```python
from build123d import *

# Parameters (mm, degrees)
BOSS_EXTRUDE2_DEPTH   = 21.844
BOSS_EXTRUDE2_2_DEPTH = 21.844
SKETCH3_W             = 4.1275
SKETCH3_H             = 39.7002
BOSS_EXTRUDE3_DEPTH   = 1.6002
SKETCH4_W             = 1.6002
SKETCH4_H             = 39.7002
BOSS_EXTRUDE4_DEPTH   = 6.5532
SKETCH5_W             = 23.4442
SKETCH5_H             = 39.7002
BOSS_EXTRUDE5_DEPTH   = 1.6002
BOSS_EXTRUDE6_DEPTH   = 4.7752
SKETCH7_W             = 21.844
SKETCH7_H             = 27.9146
CUT_EXTRUDE1_DEPTH    = 6.35


with BuildPart() as part:
    # Sketch2 → Boss-Extrude2 (new body)
    with BuildSketch(Plane(origin=(0, 0, 0), x_dir=(0, 0, -1), z_dir=(1, 0, 0))):
        Polygon((-8.001, 19.8501), (-8.001, 16.4973), (-6.4135, 16.4973), (-6.4135, 13.9573), (-10.541, 13.9573), (-10.541, 19.8501), align=None)
    extrude(amount=BOSS_EXTRUDE2_DEPTH)



with BuildPart() as body_2:
    # Sketch2 → Boss-Extrude2 2 (new body)
    with BuildSketch(Plane(origin=(0, 0, 0), x_dir=(0, 0, -1), z_dir=(1, 0, 0))):
        Polygon((-6.4135, -16.4973), (-6.4135, -13.9573), (-10.541, -13.9573), (-10.541, -19.8501), (-8.001, -19.8501), (-8.001, -16.4973), align=None)
    extrude(amount=BOSS_EXTRUDE2_2_DEPTH)


with BuildPart() as part_1:
    add(part.part)

    add(body_2.part)  # Boss-Extrude3 merges body 2
    # Sketch3 → Boss-Extrude3 (add)
    with BuildSketch(Plane.ZY):
        with Locations((8.47725, 0)):
            Rectangle(SKETCH3_W, SKETCH3_H)
    extrude(amount=BOSS_EXTRUDE3_DEPTH)

    # Sketch4 → Boss-Extrude4 (add)
    with BuildSketch(Plane(origin=(0, 0, 6.4135), x_dir=(-1, 0, 0), z_dir=(0, 0, -1))):
        with Locations((0.8001, 0)):
            Rectangle(SKETCH4_W, SKETCH4_H)
    extrude(amount=BOSS_EXTRUDE4_DEPTH)

    # Sketch5 → Boss-Extrude5 (add)
    with BuildSketch(Plane(origin=(0, 0, -0.1397), x_dir=(-1, 0, 0), z_dir=(0, 0, -1))):
        with Locations((-10.1219, 0)):
            Rectangle(SKETCH5_W, SKETCH5_H)
    extrude(amount=BOSS_EXTRUDE5_DEPTH)

    # Sketch6 → Boss-Extrude6 (add)
    with BuildSketch(Plane(origin=(0, 19.8501, 0), x_dir=(1, 0, 0), z_dir=(0, 1, 0))):
        Polygon((21.844, -8.001), (0, -8.001), (0, 0.1397), (21.844, 0.1397), (21.844, 1.7399), (-1.6002, 1.7399), (-1.6002, -10.541), (21.844, -10.541), align=None)
    boss_extrude6 = extrude(amount=BOSS_EXTRUDE6_DEPTH)

    # Mirror1: Boss-Extrude6 across plane
    add(boss_extrude6.mirror(Plane.ZX))

    # Sketch7 → Cut-Extrude1 (cut)
    with BuildSketch(Plane.XY.offset(-0.1397)):
        with Locations((10.922, 0)):
            Rectangle(SKETCH7_W, SKETCH7_H)
    extrude(amount=-CUT_EXTRUDE1_DEPTH, mode=Mode.SUBTRACT)


solid = part_1.part
```
Part model, mm, in its own coordinate system. A direction names the side the tool comes from. Coordinates: 2 decimals unless noted, no trailing zeros. Order: outer loops, then holes, each group sorted by start corner. A loop starts at its lowest first (then second) coordinate and runs counter-clockwise, first axis right, second up. Notation, with made-up numbers: (-17, 52) - (-2, 52) arc R24 cw to (-2, 90) - close; hole circle Ø3 at (30.5, 2). An arc over 180 degrees is marked (long way). Return JSON: item names as keys, results as strings. Group by question number.
Item 1: Pull direction Z, two halves, no side cores. Call faces 6 (the face through (-0.5, 0.3, 10.541)), 7 (the face through (11, 15, 6.413)), 8 (the face through (11, 13.957, 8)): pulls with the +Z half, pulls with the -Z half, needs draft (parallel to the pull), parting line crosses it, or undercut.
Item 2: Cut at B-B (y = -15.5). List the corners of the cut face in (x, z).
Item 3: Which spindle directions (+Z, -Z, +X, -X, +Y, -Y) get a long thin tool onto all of the face, cutting with end or side? Do faces 1 (the face through (11, 16.497, 7)), 2 (the face through (11, -19, -0.14)), 3 (the face through (11, -16.497, 7)), 4 (the face through (11, 13.957, -1)), 5 (the face through (21.844, -19, 9)). Say none if no direction does.
Item 4: Cut at D-D (y = -9.5). List the corners of the cut face in (x, z).
Item 5: Cut at C-C (z = -0.75). List the corners of the cut face in (x, y), plus the area to 3 significant figures.
Item 6: Pin check, flat tips, straight feed: pin 1 (3 mm diameter, centred on x = 5.5, z = 5.5, fed in from -Y); pin 2 (12 mm diameter, centred on x = 12.5, y = -5.5, fed in from +Z); pin 3 (0.8 mm diameter, centred on x = 16, z = 7, fed in from +Y). Stop position of each tip, or through.
Item 7: Drill centre lines: probe 1 along Y at (x, z) = (15.5, 7); probe 2 along Z at (x, y) = (4, -14); probe 3 along Z at (x, y) = (17.5, 21). Where is each one in solid material? Low to high. Write a range as from..to.
Item 8: Cut at A-A (x = 3.25). List the corners of the cut face in (y, z).
Check values:
{
 "1": {"face 6": "pulls with the +Z half", "face 7": "undercut", "face 8": "needs draft"},
 "2": {"outline": "(-1.6, -1.74) - (21.84, -1.74) - (21.84, -0.14) - (0, -0.14) - (0, 6.41) - (21.84, 6.41) - (21.84, 10.54) - (-1.6, 10.54) - close"},
 "3": {"face 1": "+X, +Y", "face 2": "+X, +Y, -Y", "face 3": "+X, -Y", "face 4": "+Z, -Z, +X", "face 5": "+Z, -Z, +X, +Y, -Y"},
 "4": {"outline": "(-1.6, -1.74) - (0, -1.74) - (0, 10.54) - (-1.6, 10.54) - close"},
 "5": {"outline": "(-1.6, -24.63) - (21.84, -24.63) - (21.84, -13.96) - (0, -13.96) - (0, 13.96) - (21.84, 13.96) - (21.84, 24.63) - (-1.6, 24.63) - close", "area": "545 mm2"},
 "6": {"pin 1": "stops at y = -16.5", "pin 2": "passes through", "pin 3": "stops at y = 16.5"},
 "7": {"probe 1": "y = -16.5..-13.96, 13.96..16.5", "probe 2": "z = -1.74..-0.14, 6.41..10.54", "probe 3": "z = -1.74..-0.14, 8..10.54"},
 "8": {"outline": "(-24.63, -1.74) - (-13.96, -1.74) - (-13.96, -0.14) - (-24.63, -0.14) - close; (-24.63, 8) - (-16.5, 8) - (-16.5, 6.41) - (-13.96, 6.41) - (-13.96, 10.54) - (-24.63, 10.54) - close; (13.96, -1.74) - (24.63, -1.74) - (24.63, -0.14) - (13.96, -0.14) - close; (13.96, 6.41) - (16.5, 6.41) - (16.5, 8) - (24.63, 8) - (24.63, 10.54) - (13.96, 10.54) - close"}
}
